```python
from build123d import *

# Parameters (mm, degrees)
F0_W     = 32.809374243
F0_H     = 24.5
F0_R     = 9.25
F1_DEPTH = 5
F2_W     = 5
F2_H     = 24.5
F3_DEPTH = 15
F5_DEPTH = 3
F6_W     = 14
F6_H     = 3.2
F7_DEPTH = 25
F8_R     = 1
F9_R     = 3


# Not quite as in the source:
# - a pattern or mirror of a feature is missing from the dataset's text; its kind, count and spacing are read off the source's solid


with BuildPart() as f1:
    # F0 (on Top) → F1 (new body)
    with BuildSketch(Plane.XY):
        with Locations((-4.1546871215, 0)):
            Rectangle(F0_W, F0_H)
        Circle(F0_R, mode=Mode.SUBTRACT)
    extrude(amount=F1_DEPTH)

    # F2 (on face) → F3 (join)
    with BuildSketch(Plane.XY.offset(5)):
        with Locations((-18.059374243, 0)):
            Rectangle(F2_W, F2_H)
    extrude(amount=F3_DEPTH)

    # F4 (on face) → F5 (join)
    with BuildSketch(Plane.XZ.offset(12.25)):
        Polygon((-8.5921417922, 5), (-15.559374243, 18.1631296873), (-15.559374243, 5), align=None)
    f5 = extrude(amount=-F5_DEPTH)

    # F5_copies: F5 across plane
    add(f5.mirror(Plane.ZX))

    # F6 (on face) → F7 (cut)
    with BuildSketch(Plane.YZ.offset(-15.559374243)):
        with Locations((0, 14.1660655677)):
            Rectangle(F6_W, F6_H)
    extrude(amount=-F7_DEPTH, mode=Mode.SUBTRACT)

    # F8
    f8_edges = [f1.edges().sort_by_distance(p)[0] for p in [
        (-18.059374, 7, 12.566066),
        (-18.059374, 7, 15.766066),
        (-18.059374, -7, 12.566066),
        (-18.059374, -7, 15.766066),
    ]]
    fillet(f8_edges, radius=F8_R)

    # F9
    f9_edges = [f1.edges().sort_by_distance(p)[0] for p in [
        (12.25, -12.25, 2.5),
        (12.25, 12.25, 2.5),
    ]]
    fillet(f9_edges, radius=F9_R)


solid = f1.part
```
Here's how the part is built. I have some questions about the finished solid (model axes, mm). A direction names the side the tool comes from. Coordinates: 2 decimals unless noted, no trailing zeros. Write each loop counter-clockwise with the first axis right and the second up, starting at its lowest first coordinate (ties: lowest second). Pieces come first, ordered by that corner, then holes. Notation, with made-up numbers: M 7,62.25 L 60,62.25 A21 cw 60,87.25 Z; hole C 49.5,39.5 d3. An arc over 180 degrees is marked long. Answer as CSV lines item,"result". Start each with the question number.
Q1. For faces 1 (the flat face through (-18, 0, 12.566)), 2 (the flat face through (-14, -9.25, 9)), 3 (the flat face through (-12.027, 10.771, 11.489)), which set-ups out of +Z, -Z, +X, -X, +Y, -Y let a thin tool reach every point of the face, with its end or its side?
Q2. Suppose I cut it at A-A, the plane x = -17. List the corners of the cut face in (y, z) for me.
Q3. Will these pins go through, and if not, where does the flat tip stop? pin 1 Ø3.5 at (x, z) = (-10.5, 12.5) entering from -Y; pin 2 Ø5 at (y, z) = (-5, 9) entering from +X.
Q4. Suppose I cut it at D-D, the plane z = 3.5. List the corners of the cut face in (x, y) for me, then the cut area to 3 significant figures.
Q5. I need wall thicknesses on probe 1 along Z at (x, y) = (-17.5, -6); probe 2 along Y at (x, z) = (0, 2.8); probe 3 along X at (y, z) = (9, 14.5). Which ranges of each line are inside material? Lowest first, please. Write a range as [from, to].
Q6. Suppose I cut it at B-B, the plane y = 0. List the corners of the cut face in (x, z) for me, then the cut area to 3 significant figures.
Q7. Suppose I cut it at C-C, the plane y = 8.5. List the corners of the cut face in (x, z) for me, then the cut area to 3 significant figures.
Q8. If we mould it in two halves opening along Y, with no side actions, what happens to faces 4 (the cylindrical face through (-18.094, 6.715, 12.867)), 5 (the cylindrical face through (-18.094, -6.715, 12.867)), 6 (the flat face through (12.25, 0, 2)), 7 (the cylindrical face through (11.35, -11.39, 2.54))? For each: pulls with the +Y half, pulls with the -Y half, needs draft (parallel to the pull), parting line crosses it, or undercut.
Entries:
1,face 1,"+X, -X"
1,face 2,"+Z, +X"
1,face 3,"+Z, +X, +Y, -Y"
2,outline,"M -12.25,0 L 12.25,0 L 12.25,20 L -12.25,20 Z; hole M -7,13.57 A1 ccw -6,12.57 L 6,12.57 A1 ccw 7,13.57 L 7,14.77 A1 ccw 6,15.77 L -6,15.77 A1 ccw -7,14.77 Z"
3,pin 1,"passes through"
3,pin 2,"stops at x = -15.56"
4,outline,"M -20.56,-12.25 L 9.25,-12.25 A3 ccw 12.25,-9.25 L 12.25,9.25 A3 ccw 9.25,12.25 L -20.56,12.25 Z; hole C 0,0 d18.5"
4,area,"531 mm²"
5,probe 1,"z = [0, 12.57], [15.77, 20]"
5,probe 2,"y = [-12.25, -9.25], [9.25, 12.25]"
5,probe 3,"x = [-20.56, -15.56]"
6,outline,"M -20.56,0 L -9.25,0 L -9.25,5 L -15.56,5 L -15.56,12.57 L -20.56,12.57 Z; M -20.56,15.77 L -15.56,15.77 L -15.56,20 L -20.56,20 Z; M 9.25,0 L 12.25,0 L 12.25,5 L 9.25,5 Z"
6,area,"131 mm²"
7,outline,"M -20.56,0 L -3.65,0 L -3.65,5 L -15.56,5 L -15.56,20 L -20.56,20 Z; M 3.65,0 L 12.25,0 L 12.25,5 L 3.65,5 Z"
7,area,"203 mm²"
8,face 4,"undercut"
8,face 5,"undercut"
8,face 6,"needs draft"
8,face 7,"pulls with the -Y half"
